```python
from build123d import *

# Parameters (mm, degrees)
F1_DEPTH = 3


with BuildPart() as f1:
    # F0 (on Right) → F1 (new body)
    with BuildSketch(Plane.YZ):
        Polygon((33.589474, -20.788582), (50.589474, -20.788582), (50.589474, -13.788582), (53.589474, -13.788582), (53.589474, -3.788582), (50.589474, -3.788582), (50.589474, 3.211418), (53.589474, 3.211418), (53.589474, 13.211418), (50.589474, 13.211418), (50.589474, 20.211418), (33.589474, 20.211418), (33.589474, 23.211418), (23.589474, 23.211418), (23.589474, 20.211418), (14.589474, 20.211418), (14.589474, 16.711418), (15.698332, 16.711418), (15.698332, 14.711418), (14.589474, 14.711418), (14.589474, 8.211418), (12.80719, 8.211418), (12.80719, 14.711418), (11.698332, 14.711418), (11.698332, 16.711418), (12.80719, 16.711418), (12.80719, 20.12675), (3.589474, 20.211418), (3.589474, 23.211418), (-6.410526, 23.211418), (-6.410526, 20.211418), (-15.628242, 20.211418), (-15.628242, 16.711418), (-14.519384, 16.711418), (-14.519384, 14.711418), (-15.628242, 14.711418), (-15.628242, 8.211418), (-17.410526, 8.211418), (-17.410526, 14.711418), (-18.519384, 14.711418), (-18.519384, 16.711418), (-17.410526, 16.711418), (-17.410526, 20.211418), (-26.410526, 20.211418), (-26.410526, 23.211418), (-36.410526, 23.211418), (-36.410526, 20.211418), (-53.410526, 20.211418), (-53.410526, 13.211418), (-56.410526, 13.211418), (-56.410526, 3.211418), (-53.410526, 3.211418), (-53.410526, -3.788582), (-56.410526, -3.788582), (-56.410526, -13.788582), (-53.410526, -13.788582), (-53.410526, -20.788582), (-36.410526, -20.788582), (-36.410526, -23.788582), (-26.410526, -23.788582), (-26.410526, -20.788582), (-17.410526, -20.788582), (-17.410526, -14.288582), (-18.410526, -14.288582), (-18.410526, -12.288582), (-17.410526, -12.288582), (-17.410526, -8.788582), (-15.410526, -8.788582), (-15.410526, -12.288582), (-14.410526, -12.288582), (-14.410526, -14.288582), (-15.410526, -14.288582), (-15.410526, -20.788582), (-6.410526, -20.788582), (-6.410526, -23.788582), (3.589474, -23.788582), (3.589474, -20.788582), (12.589474, -20.788582), (12.589474, -14.288582), (11.589474, -14.288582), (11.589474, -12.288582), (12.589474, -12.288582), (12.589474, -8.788582), (14.589474, -8.788582), (14.589474, -12.288582), (15.589474, -12.288582), (15.589474, -14.288582), (14.589474, -14.288582), (14.589474, -20.788582), (23.589474, -20.788582), (23.589474, -23.788582), (33.589474, -23.788582), align=None)
    extrude(amount=F1_DEPTH)


solid = f1.part
```
Read the model definition and answer for the solid it produces. Units are mm, in the model's axes. A direction names the side the tool comes from. Coordinates: 2 decimals unless noted, no trailing zeros. Order: outer loops, then holes, each group sorted by start corner. A loop starts at its lowest first (then second) coordinate and runs counter-clockwise, first axis right, second up. Notation, with made-up numbers: (4, 7) - (45, 7) arc R12 ccw to (45, 14) - close; hole circle Ø3 at (2.25, 31). An arc over 180 degrees is marked (long way). Answer as a JSON object with one key per item and string values. Group by question number.
Item 1: The mould has two halves that part along Z. Classify faces 5 (the face through (1, 52, 3.211)), 6 (the face through (1, -26.411, 22)), 7 (the face through (1, -16, -8.789)): +Z half, -Z half, draft (parallel to the pull), parting line (faces both ways), or undercut.
Item 2: Section C-C (y = -11) is taken. Give the vertices of the cut face in (x, z), plus the area to 3 significant figures.
Item 3: A tool of negligible diameter and unlimited length cuts with its end or side. For faces 1 (the face through (1, 14.589, -11)), 2 (the face through (1, 33.589, 22)), 3 (the face through (1, -11, 20.211)), 4 (the face through (1, 50.589, -17)), from which of +Z, -Z, +X, -X, +Y, -Y can it reach the whole face along a straight path? Write none if from no direction.
Item 4: Consider probe 1 along Y at (x, z) = (0.6, 21.5); probe 2 along Y at (x, z) = (2.2, 11); probe 3 along Z at (x, y) = (2.8, -15). Determine where each line is inside the solid, lowest interval first. Write a range as from..to.
Item 5: Section A-A (z = -18) is taken. Give the vertices of the cut face in (x, y), plus the area to 3 significant figures.
Item 6: Flat-ended cylindrical pins translate along their axes: P1, Ø1.5, axis at x = 1, y = -54.5, coming from the -Z side; P2, Ø1.6, axis at x = 2, z = 15.5, coming from the -Y side; P3, Ø1.2, axis at x = 1.5, y = -18, coming from the +Z side. Find the tip coordinate at first contact, or state that the pin passes through.
Item 7: Section B-B (z = 11) is taken. Give the vertices of the cut face in (x, y), plus the area to 3 significant figures.
Results are:
{
 "1": {"face 5": "undercut", "face 6": "draft", "face 7": "-Z half"},
 "2": {"outline": "(0, -20.79) - (3, -20.79) - (3, 20.21) - (0, 20.21) - close", "area": "123 mm^2"},
 "3": {"face 1": "-Z, +X, -X", "face 2": "+Z, +X, -X, +Y", "face 3": "+Z, +X, -X", "face 4": "-Z, +X, -X, +Y"},
 "4": {"probe 1": "y = -36.41..-26.41, -6.41..3.59, 23.59..33.59", "probe 2": "y = -56.41..-17.41, -15.63..12.81, 14.59..53.59", "probe 3": "z = -20.79..-14.29, -12.29..14.71, 16.71..20.21"},
 "5": {"outline": "(0, -53.41) - (3, -53.41) - (3, -17.41) - (0, -17.41) - close; (0, -15.41) - (3, -15.41) - (3, 12.59) - (0, 12.59) - close; (0, 14.59) - (3, 14.59) - (3, 50.59) - (0, 50.59) - close", "area": "300 mm^2"},
 "6": {"P1": "stops at z = -13.79", "P2": "stops at y = -53.41", "P3": "stops at z = 20.21"},
 "7": {"outline": "(0, -56.41) - (3, -56.41) - (3, -17.41) - (0, -17.41) - close; (0, -15.63) - (3, -15.63) - (3, 12.81) - (0, 12.81) - close; (0, 14.59) - (3, 14.59) - (3, 53.59) - (0, 53.59) - close", "area": "319 mm^2"}
}
